Check sheet for the modelled part. Datum: model origin and axes. Units: mm. Face numbers are marked on the shaded views. A direction names the side the tool comes from. Give positions to 0.01 mm unless a question says otherwise; leave off trailing zeros. Loops run counter-clockwise (first coordinate to the right, second up) from the corner with the lowest first, then second, coordinate; pieces in that order, holes last. Notation, with made-up numbers: (-17.5, 39) - (39.5, 39) arc R14 cw to (39.5, 51) - close; hole circle Ø10 at (-18, 16). An arc over 180 degrees is marked (long way). Use CSV: the item, a comma, the result in double quotes.
Autodesk Inventor part; units mm, degrees
ref_plane "Work Plane1" through (0, 39, 0) normal (0, 1, 0) x (1, 0, 0)
ref_plane "YZ Plane" through (0, 0, 0) normal (1, 0, 0) x (0, 1, 0)
ref_plane "XZ Plane" through (0, 0, 0) normal (0, 1, 0) x (-1, 0, 0)
sketch "Sketch1" plane through (0, 0, 0) normal (0, 1, 0) x (-1, 0, 0)
  circle A0 centre (0, 0) radius 1
  dimension "d0" = 2
extrude "Extrusion1" add sketch "Sketch1" along normal blind 40
sketch "Sketch2" plane through (0, 40, 0) normal (0, 1, 0) x (1, 0, 0)
  circle A0 centre (0, 0) radius 2.1
  dimension "d3" = 4.2
ref_plane "Work Plane1" through (0, 39, 0) normal (0, 1, 0) x (1, 0, 0)
sketch "Sketch3" plane through (0, 39, 0) normal (0, 1, 0) x (1, 0, 0)
  circle A0 centre (0, 0) radius 1
loft "Loft1" add profiles "Sketch3", "Sketch2"
sketch "Sketch4" plane through (0, 40, 0) normal (0, 1, 0) x (1, 0, 0)
  line L0 (-1.7, -0.3) -> (1.7, -0.3)
  line L1 (1.7, -0.3) -> (1.7, 0.3)
  line L2 (1.7, 0.3) -> (-1.7, 0.3)
  line L3 (-1.7, 0.3) -> (-1.7, -0.3)
  line L4 (-0.3, -1.7) -> (0.3, -1.7)
  line L5 (0.3, -1.7) -> (0.3, 1.7)
  line L6 (0.3, 1.7) -> (-0.3, 1.7)
  line L7 (-0.3, 1.7) -> (-0.3, -1.7)
  point P0 (0, 0)
  point P1 (-1.7, 0)
  point P2 (0, -1.7)
  point P3 (0, -0.3)
  point P4 (0.3, 0)
  point P5 (-0.3, -0.3)
  point P6 (0.3, -0.3)
  point P7 (0.3, 0.3)
  point P8 (-0.3, 0.3)
  dimension "d9" = 3.4
  dimension "d10" = 3.4
  dimension "d11" = 0.6
  dimension "d12" = 0.6
extrude "Extrusion2" cut sketch "Sketch4" against normal blind 0.3
chamfer "Chamfer1" distance 0.3 distance2 1 1 edges at (1.7, 39.7, 0) measured on face at (1.7, 39.9, 0.1)
chamfer "Chamfer2" distance 0.3 distance2 1 1 edges at (0, 39.7, 1.7) measured on face at (-0.1, 39.9, 1.7)
chamfer "Chamfer3" distance 0.3 distance2 1 1 edges at (-1.7, 39.7, 0) measured on face at (-1.7, 39.9, -0.1)
chamfer "Chamfer4" distance 0.3 distance2 1 1 edges at (0, 39.7, -1.7) measured on face at (0.1, 39.9, -1.7)
fillet "Fillet1" radius 0.4 4 edges at (0.3, 39.85, 0.3) (-0.3, 39.85, 0.3) (0.3, 39.85, -0.3) (-0.3, 39.85, -0.3)
thread "Thread1"
equation "\"d12\" = d11"
properties part number "m2_40mm" material "Stainless Steel"
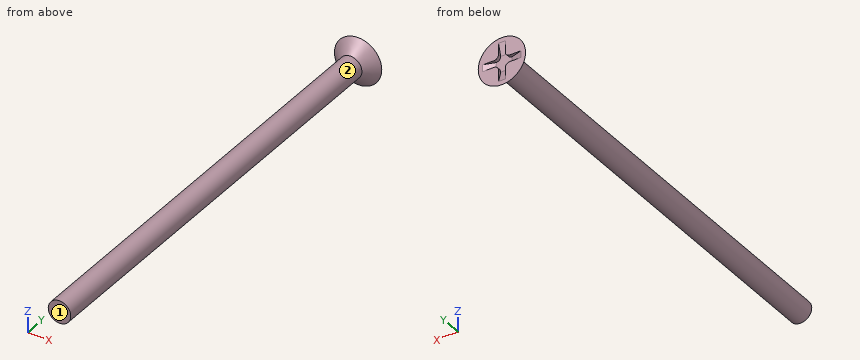
1. Go/stop test with a flat-tipped pin: pin 1 Ø0.7 at (x, z) = (0, 0) entering from +Y. Record where the tip stops, or that it passes through.
Completed:
pin 1,"stops at y = 39.7"
2. Sectioned sample at A-A, the plane y = 34. Record the boundary of the cut face in (x, z).
Completed:
outline,"circle Ø2 at (0, 0)"
3. Scan lines: line 1 along Y through (x, z) = (-0.35, 0); line 2 along Y through (x, z) = (0.4, -0.95); line 3 along Z through (x, y) = (0.25, 26). Record each from-to range of solid material in increasing order.
Completed:
line 1,"y = 0 to 39.7"
line 2,"y = 39.03 to 40"
line 3,"z = -0.97 to 0.97"
4. Set-up check for the marked faces 1 and 2: record each of +Z, -Z, +X, -X, +Y, -Y from which the full face is reachable in a straight line by a thin tool's end or side.
Completed:
face 1,"+Z, -Z, +X, -X, -Y"
face 2,"-Y"
